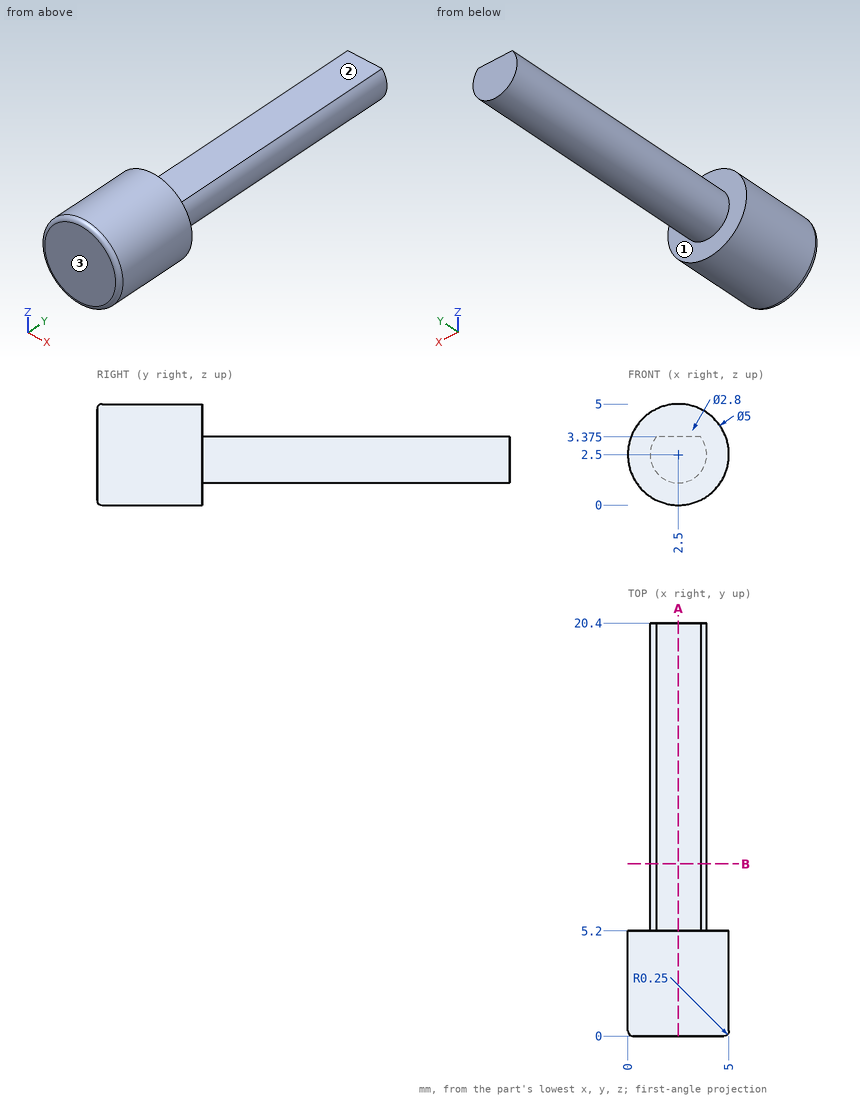
Here's the drawing with two shaded views (mm, measured from the low corner). I have some questions. A direction names the side the tool comes from. Give positions to 0.01 mm unless a question says otherwise; leave off trailing zeros. Write each loop counter-clockwise with the first axis right and the second up, starting at its lowest first coordinate (ties: lowest second). Pieces come first, ordered by that corner, then holes. Notation, with made-up numbers: (64, 67.5) -> (118, 67.5) arc R28 ccw to (118, 88.5) -> close; hole circle Ø9 at (-32.5, 73). An arc over 180 degrees is marked (long way). Answer as a JSON object with one key per item and string values. Group by question number.
Item 1: For the marked faces 1, 2 and 3, which set-ups out of +Z, -Z, +X, -X, +Y, -Y let a thin tool reach every point of the face, with its end or its side?
Item 2: Please list where these lines run through material, in increasing order: line 1 (Y direction, x = 3.15, z = 4.05); line 2 (Z direction, x = 2.35, y = 4.75); line 3 (Z direction, x = 2.95, y = 11.75) (3 decimals). Write a range as [from, to].
Item 3: Suppose I cut it at B-B (y = 8.5). Please give me the cut outline in (x, z) (3 decimals), plus the area to 3 significant figures.
Item 4: I'm going to push flat-ended pins straight in: P1, Ø1, axis at y = 8, z = 2, coming from the +X side; P2, Ø1.1, axis at x = 2.5, y = 9.5, coming from the +Z side (3 decimals); P3, Ø2, axis at x = 4.5, y = 11, coming from the -Z side. Where does each tip first touch, or does it pass through?
Item 5: Suppose I cut it at A-A (x = 2.5). Please give me the cut outline in (y, z) (3 decimals), plus the area to 3 significant figures.
Findings:
{
 "1": {"face 1": "+Y", "face 2": "+Z, +X, -X, +Y", "face 3": "+Z, -Z, +X, -X, -Y"},
 "2": {"line 1": "y = [0, 5.2]", "line 2": "z = [0, 5]", "line 3": "z = [1.174, 3.375]"},
 "3": {"outline": "(1.407, 3.375) arc R1.4 ccw (long way) to (3.593, 3.375) -> close", "area": "5.36 mm²"},
 "4": {"P1": "stops at x = 3.9", "P2": "stops at z = 3.375", "P3": "stops at z = 1.52"},
 "5": {"outline": "(0, 0.25) arc R0.25 ccw to (0.25, 0) -> (5.2, 0) -> (5.2, 1.1) -> (20.4, 1.1) -> (20.4, 3.375) -> (5.2, 3.375) -> (5.2, 5) -> (0.25, 5) arc R0.25 ccw to (0, 4.75) -> close", "area": "60.6 mm²"}
}
